Source: CAD feature listing. Evaluate the final solid. Frame: model axes, mm. Face numbers are marked on the shaded views. A direction names the side the tool comes from. Give positions to 0.01 mm unless a question says otherwise; leave off trailing zeros. Order: outer loops, then holes, each group sorted by start corner. A loop starts at its lowest first (then second) coordinate and runs counter-clockwise, first axis right, second up.
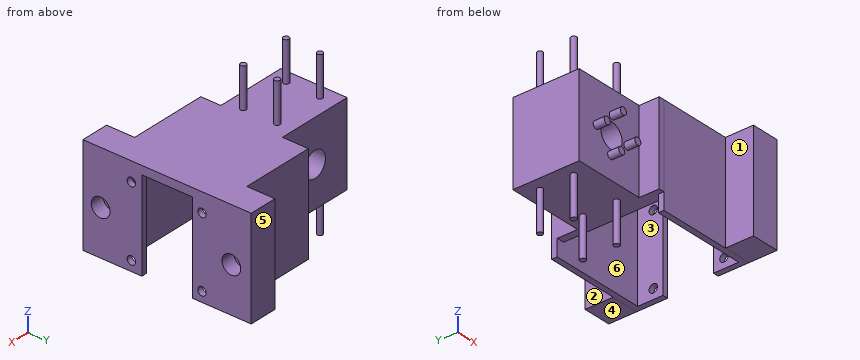
```python
from build123d import *

# Parameters (mm, degrees)
SKETCH1_W            = 34.7
SKETCH1_H            = 30
BOSS_EXTRUDE1_DEPTH  = 37.282
SKETCH2_R            = 1.27
BOSS_EXTRUDE2_DEPTH  = 18
SKETCH4_R            = 5.715
CUT_EXTRUDE1_DEPTH   = 31
SKETCH5_R            = 1.625
BOSS_EXTRUDE4_DEPTH  = 5
SKETCH6_R            = 1.27
BOSS_EXTRUDE5_DEPTH  = 18
SKETCH8_W            = 3.81
SKETCH8_H            = 50.8
BOSS_EXTRUDE6_DEPTH  = 45.72
BOSS_EXTRUDE7_DEPTH  = 41.000001
CUT_EXTRUDE2_REACH   = 82.42
SKETCH10_R           = 1.905
SKETCH11_W           = 12.7
SKETCH11_H           = 44.810000611
BOSS_EXTRUDE8_DEPTH  = 12.7
SKETCH12_W           = 12.7
SKETCH12_H           = 44.810000611
BOSS_EXTRUDE9_DEPTH  = 12.7
SKETCH13_R           = 4.25
CUT_EXTRUDE3_DEPTH   = 6.35
SKETCH17_W           = 3.43592392
SKETCH17_H           = 45.72
BOSS_EXTRUDE12_DEPTH = 33.472
SKETCH16_W           = 2.5
SKETCH16_H           = 37.282
BOSS_EXTRUDE11_DEPTH = 9.076061


with BuildPart() as part:
    # Sketch1 → Boss-Extrude1 (new body)
    with BuildSketch(Plane(origin=(0, 0, -264.675), x_dir=(-1, 0, 0), z_dir=(0, 0, -1))):
        with Locations((-46.026450848, -396.896376681)):
            Rectangle(SKETCH1_W, SKETCH1_H)
    extrude(amount=BOSS_EXTRUDE1_DEPTH)

    # Sketch2 → Boss-Extrude2 (add)
    with BuildSketch(Plane.XY.offset(-264.675)):
        with Locations((34.526450848, -389.246376681)):
            Circle(SKETCH2_R)
        with Locations((57.526450848, -389.246376681)):
            Circle(SKETCH2_R)
        with Locations((57.526450848, -404.546376681)):
            Circle(SKETCH2_R)
        with Locations((34.526450848, -404.546376681)):
            Circle(SKETCH2_R)
    extrude(amount=BOSS_EXTRUDE2_DEPTH)

    # Sketch4 → Cut-Extrude1 (cut, through all)
    with BuildSketch(Plane(origin=(0, -381.896376681, 0), x_dir=(1, 0, 0), z_dir=(0, 1, 0))):
        with Locations((46.026450848, 283.749893694)):
            Circle(SKETCH4_R)
    extrude(amount=-CUT_EXTRUDE1_DEPTH, mode=Mode.SUBTRACT)

    # Sketch5 → Boss-Extrude4 (add)
    with BuildSketch(Plane.XZ.offset(411.896376681)):
        with Locations((46.453266338, -275.535975412)):
            Circle(SKETCH5_R)
        with Locations((54.24036913, -284.176709184)):
            Circle(SKETCH5_R)
        with Locations((45.599635358, -291.963811975)):
            Circle(SKETCH5_R)
        with Locations((37.812532567, -283.323078204)):
            Circle(SKETCH5_R)
    extrude(amount=BOSS_EXTRUDE4_DEPTH)

    # Sketch6 → Boss-Extrude5 (add)
    with BuildSketch(Plane(origin=(0, 0, -301.957), x_dir=(-1, 0, 0), z_dir=(0, 0, -1))):
        with Locations((-57.526450848, -389.246376681)):
            Circle(SKETCH6_R)
        with Locations((-34.526450848, -389.246376681)):
            Circle(SKETCH6_R)
        with Locations((-34.526450848, -404.546376681)):
            Circle(SKETCH6_R)
        with Locations((-57.526450848, -404.546376681)):
            Circle(SKETCH6_R)
    extrude(amount=BOSS_EXTRUDE5_DEPTH)

    # Sketch8 → Boss-Extrude6 (add)
    with BuildSketch(Plane(origin=(63.376450848, 0, 0), x_dir=(0, 0, -1), z_dir=(1, 0, 0))):
        with Locations((266.58, -395.572437442)):
            Rectangle(SKETCH8_W, SKETCH8_H)
    extrude(amount=BOSS_EXTRUDE6_DEPTH)

    # Sketch9 → Boss-Extrude7 (add)
    with BuildSketch(Plane(origin=(0, 0, -268.485), x_dir=(-1, 0, 0), z_dir=(0, 0, -1))):
        Polygon((-109.096450848, -370.172437442), (-63.376450848, -370.172437442), (-63.376450848, -372.712437442), (-106.556450848, -372.712437442), (-106.556450848, -384.142437442), (-109.096450848, -384.142437442), (-109.096450848, -372.712437442), align=None)
        Polygon((-109.096450848, -420.972437442), (-63.376450848, -420.972437442), (-63.376450848, -418.432437442), (-106.556450848, -418.432437442), (-106.556450848, -407.002437442), (-109.096450848, -407.002437442), (-109.096450848, -418.432437442), align=None)
    extrude(amount=BOSS_EXTRUDE7_DEPTH)

    # Sketch10 → Cut-Extrude2 (cut, up to next)
    with BuildSketch(Plane(origin=(109.096450848, 0, 0), x_dir=(0, 0, -1), z_dir=(1, 0, 0)), mode=Mode.PRIVATE) as cut_extrude2_sk1:
        with Locations((304.963451053, -379.773986799)):
            Circle(SKETCH10_R)
    cut_extrude2_tool1 = extrude(cut_extrude2_sk1.sketch, amount=-CUT_EXTRUDE2_REACH, mode=Mode.PRIVATE) & part.part
    add(cut_extrude2_tool1.solids().sort_by_distance((109.096451, -379.773987, -304.963451))[0], mode=Mode.SUBTRACT)
    # Sketch10 → Cut-Extrude2 (cut, up to next)
    with BuildSketch(Plane(origin=(109.096450848, 0, 0), x_dir=(0, 0, -1), z_dir=(1, 0, 0)), mode=Mode.PRIVATE) as cut_extrude2_sk2:
        with Locations((304.941901697, -411.752437852)):
            Circle(SKETCH10_R)
    cut_extrude2_tool2 = extrude(cut_extrude2_sk2.sketch, amount=-CUT_EXTRUDE2_REACH, mode=Mode.PRIVATE) & part.part
    add(cut_extrude2_tool2.solids().sort_by_distance((109.096451, -411.752438, -304.941902))[0], mode=Mode.SUBTRACT)
    # Sketch10 → Cut-Extrude2 (cut, up to next)
    with BuildSketch(Plane(origin=(109.096450848, 0, 0), x_dir=(0, 0, -1), z_dir=(1, 0, 0)), mode=Mode.PRIVATE) as cut_extrude2_sk3:
        with Locations((273.239000003, -379.752437442)):
            Circle(SKETCH10_R)
    cut_extrude2_tool3 = extrude(cut_extrude2_sk3.sketch, amount=-CUT_EXTRUDE2_REACH, mode=Mode.PRIVATE) & part.part
    add(cut_extrude2_tool3.solids().sort_by_distance((109.096451, -379.752437, -273.239))[0], mode=Mode.SUBTRACT)
    # Sketch10 → Cut-Extrude2 (cut, up to next)
    with BuildSketch(Plane(origin=(109.096450848, 0, 0), x_dir=(0, 0, -1), z_dir=(1, 0, 0)), mode=Mode.PRIVATE) as cut_extrude2_sk4:
        with Locations((273.221901697, -411.730888495)):
            Circle(SKETCH10_R)
    cut_extrude2_tool4 = extrude(cut_extrude2_sk4.sketch, amount=-CUT_EXTRUDE2_REACH, mode=Mode.PRIVATE) & part.part
    add(cut_extrude2_tool4.solids().sort_by_distance((109.096451, -411.730888, -273.221902))[0], mode=Mode.SUBTRACT)

    # Sketch11 → Boss-Extrude8 (add)
    with BuildSketch(Plane(origin=(0, -370.172437442, 0), x_dir=(1, 0, 0), z_dir=(0, 1, 0))):
        with Locations((102.746450848, 287.080000305)):
            Rectangle(SKETCH11_W, SKETCH11_H)
    extrude(amount=BOSS_EXTRUDE8_DEPTH)

    # Sketch12 → Boss-Extrude9 (add)
    with BuildSketch(Plane.XZ.offset(420.972437442)):
        with Locations((102.746450848, -287.080000305)):
            Rectangle(SKETCH12_W, SKETCH12_H)
    extrude(amount=BOSS_EXTRUDE9_DEPTH)

    # Sketch13 → Cut-Extrude3 (cut)
    with BuildSketch(Plane(origin=(109.096450848, 0, 0), x_dir=(0, 0, -1), z_dir=(1, 0, 0))):
        with Locations((288.985000522, -366.472437442)):
            Circle(SKETCH13_R)
        with Locations((288.985000522, -425.654437442)):
            Circle(SKETCH13_R)
    extrude(amount=-CUT_EXTRUDE3_DEPTH, mode=Mode.SUBTRACT)

    # Sketch17 → Boss-Extrude12 (add)
    with BuildSketch(Plane(origin=(0, 0, -268.485), x_dir=(-1, 0, 0), z_dir=(0, 0, -1))):
        with Locations((-65.094412808, -395.572437442)):
            Rectangle(SKETCH17_W, SKETCH17_H)
    extrude(amount=BOSS_EXTRUDE12_DEPTH)

    # Sketch16 → Boss-Extrude11 (add)
    with BuildSketch(Plane.XZ.offset(411.896376681)):
        with Locations((62.126450848, -283.316)):
            Rectangle(SKETCH16_W, SKETCH16_H)
    extrude(amount=BOSS_EXTRUDE11_DEPTH)


solid = part.part
```
1) Section query D-D, the plane y = -401.5. Return the cut outline in (x, z) (3 decimals).
Report:
outline: (28.676, -301.957) - (66.812, -301.957) - (66.812, -268.485) - (109.096, -268.485) - (109.096, -264.675) - (28.676, -264.675) - close; hole circle Ø11.43 at (46.026, -283.75)
2) Section query A-A, the plane z = -305. Return the cut outline in (x, y).
Report:
outline: circle Ø2.54 at (34.53, -404.55); circle Ø2.54 at (34.53, -389.25); circle Ø2.54 at (57.53, -404.55); circle Ø2.54 at (57.53, -389.25); (63.38, -420.97) - (96.4, -420.97) - (96.4, -433.67) - (109.1, -433.67) - (109.1, -413.66) - (106.56, -413.66) - (106.56, -418.43) - (63.38, -418.43) - close; (63.38, -372.71) - (106.56, -372.71) - (106.56, -377.87) - (109.1, -377.87) - (109.1, -357.47) - (96.4, -357.47) - (96.4, -370.17) - (63.38, -370.17) - close; (106.56, -409.85) - (109.1, -409.85) - (109.1, -407) - (106.56, -407) - close; (106.56, -384.14) - (109.1, -384.14) - (109.1, -381.68) - (106.56, -381.68) - close
3) Section query C-C, the plane z = -267. Return the cut outline in (x, y).
Report:
outline: (28.68, -411.9) - (60.88, -411.9) - (60.88, -420.97) - (96.4, -420.97) - (96.4, -433.67) - (109.1, -433.67) - (109.1, -357.47) - (96.4, -357.47) - (96.4, -370.17) - (63.38, -370.17) - (63.38, -381.9) - (28.68, -381.9) - close
4) Draft query along Y for the marked faces 4, 5 and 6. Return one class per face: +Y half, -Y half, draft (parallel to the pull), parting line (faces both ways), or undercut.
Report:
face 4: draft
face 5: +Y half
face 6: undercut
5) Section query B-B, the plane x = 99. Return the cut outline in (y, z) (3 decimals).
Report:
outline: (-433.672, -309.485) - (-418.432, -309.485) - (-418.432, -268.485) - (-372.712, -268.485) - (-372.712, -309.485) - (-357.472, -309.485) - (-357.472, -264.675) - (-433.672, -264.675) - close
6) Reachability of the marked faces 1, 2 and 3 from +Z, -Z, +X, -X, +Y, -Y: full face, straight path, thin tool, end or side. Return the list, or none.
Report:
face 1: +Z, -Z, -X, -Y
face 2: +Z, -Z, -X, +Y
face 3: -Z
7) Material intervals for L1, parallel to Y at x = 73, z = -269; L2, parallel to Y at x = 98, z = -302; L3, parallel to X at y = -389, z = -284, sorted ascending.
Report:
L1: y = -420.97 to -418.43, -372.71 to -370.17
L2: y = -433.67 to -418.43, -372.71 to -357.47
L3: x = 28.68 to 40.32, 51.74 to 66.81
8) Pin query (flat end, axial travel): pin 1 (6.5 mm diameter, centred on y = -363, z = -291.5, fed in from -X); pin 2 (2.5 mm diameter, centred on x = 54, z = -283.5, fed in from -Y); pin 3 (4 mm diameter, centred on y = -424.5, z = -290, fed in from +X). Return the tip coordinate at first contact, or that it passes through.
Report:
pin 1: stops at x = 96.4
pin 2: stops at y = -416.9
pin 3: stops at x = 102.75
